from build123d import *

# Parameters (mm, degrees)
F0_W     = 0.834487
F0_H     = 4.677228
F0_R     = 5.597638
F1_DEPTH = 3.2512


with BuildPart() as f1:
    # F0 (on Front) → F1 (new body)
    with BuildSketch(Plane.XZ):
        with Locations((-16.629863, -2.933552)):
            Rectangle(F0_W, F0_H)
        with BuildLine():
            Line((-17.047107, -5.272166), (-17.047107, -6.060281))
            Line((-17.047107, -6.060281), (20.092821, -6.060281))
            Line((20.092821, -6.060281), (20.092821, 16.750548))
            add(Edge.make_bspline(
                [(12.386335, 22.250686), (13.07097, 20.542209), (14.079554, 17.765705), (18.172912, 18.994402), (19.766842, 17.223716), (20.092821, 16.750548)],
                knots=[0, 0, 0, 0, 4.344221, 8.073844, 10.215903, 10.215903, 10.215903, 10.215903], degree=3))
            ThreePointArc((12.386335, 22.250686), (-0.010698, 14.235434), (-3.920062, 0))
            Line((-3.920062, 0), (-17.047107, 0))
            Line((-17.047107, 0), (-17.047107, -0.594938))
            Line((-17.047107, -0.594938), (-16.21262, -0.594938))
            Line((-16.21262, -0.594938), (-16.21262, -5.272166))
            Line((-16.21262, -5.272166), (-17.047107, -5.272166))
        make_face()
        with Locations((3.032837, 0.080925)):
            Circle(F0_R, mode=Mode.SUBTRACT)
        with BuildLine():
            add(Edge.make_bspline(
                [(12.386335, 22.250686), (13.07097, 20.542209), (14.079554, 17.765705), (18.172912, 18.994402), (19.766842, 17.223716), (20.092821, 16.750548)],
                knots=[0, 0, 0, 0, 4.344221, 8.073844, 10.215903, 10.215903, 10.215903, 10.215903], degree=3))
            Line((20.092821, 16.750548), (20.092821, 22.755181))
            ThreePointArc((20.092821, 22.755181), (16.877156, 19.526201), (13.369215, 22.435008))
            ThreePointArc((13.369215, 22.435008), (12.876662, 22.34878), (12.386335, 22.250686))
        make_face()
    extrude(amount=-F1_DEPTH)


solid = f1.part
Geometry check sheet. Reference: the model listing, model coordinates, mm. Round coordinates to 2 decimals unless told otherwise and drop trailing zeros. Loops run counter-clockwise (first coordinate to the right, second up) from the corner with the lowest first, then second, coordinate; pieces in that order, holes last.
Item 1: Cross-section at D-D on x = -8. Record the boundary of the cut face in (y, z).
Item 2: Gauge pin test, flat ends, axial feed: pin 1 (1 mm diameter, centred on x = 11, y = 2.5, fed in from +Z); pin 2 (1 mm diameter, centred on x = -10.5, y = 2, fed in from +Z); pin 3 (1 mm diameter, centred on x = 3, y = 0.5, fed in from +Z). Record the tip position at first contact, or that the pin passes through.
Item 3: Cross-section at A-A on z = 0.5. Record the boundary of the cut face in (x, y).
Item 4: Cross-section at C-C on y = 0.6. Record the boundary of the cut face in (x, z) (3 decimals), then the cut area to 3 significant figures.
Item 5: Cross-section at B-B on x = 0.5. Record the boundary of the cut face in (y, z), then the cut area to 3 significant figures.
Item 6: Mould release check, pull along Z, two halves, no side actions. Record for faces 1 (the cylindrical face through (-2.56, 1.6, 0.33)), 2 (the cylindrical face through (16.95, 1.6, 19.53)), 3 (the flat face through (5.39, 3.251, 5.35)): pulls with the +Z half, pulls with the -Z half, needs draft (parallel to the pull), parting line crosses it, or undercut.
Item 7: Thickness scan on line 1 (Z direction, x = -8, y = 1.65); line 2 (Z direction, x = -1.5, y = 1.8); line 3 (X direction, y = 2.3, z = 20.5). Record the ranges inside material, lowest first.
Answer sheet:
1. outline: (0, -6.06) - (3.25, -6.06) - (3.25, 0) - (0, 0) - close
2. pin 1: stops at z = 22.04
2. pin 2: stops at z = 0
2. pin 3: stops at z = 17.96
3. outline: (-3.96, 0) - (-2.55, 0) - (-2.55, 3.25) - (-3.96, 3.25) - close; (8.61, 0) - (20.09, 0) - (20.09, 3.25) - (8.61, 3.25) - close
4. outline: (-17.047, -6.06) - (20.093, -6.06) - (20.093, 22.755) arc R3.38 cw to (13.369, 22.435) arc R20.711 ccw to (12.386, 22.251) arc R20.71 ccw to (-3.92, 0) - (-17.047, 0) - close; hole circle Ø11.195 at (3.033, 0.081)
4. area: 566 mm2
5. outline: (0, -6.06) - (3.25, -6.06) - (3.25, -4.91) - (0, -4.91) - close; (0, 5.07) - (3.25, 5.07) - (3.25, 14.9) - (0, 14.9) - close
5. area: 35.7 mm2
6. face 1: undercut
6. face 2: pulls with the +Z half
6. face 3: needs draft
7. line 1: z = -6.06 to 0
7. line 2: z = -6.06 to -3.2, 3.37 to 11.89
7. line 3: x = 7.4 to 14.34, 19.09 to 20.09
